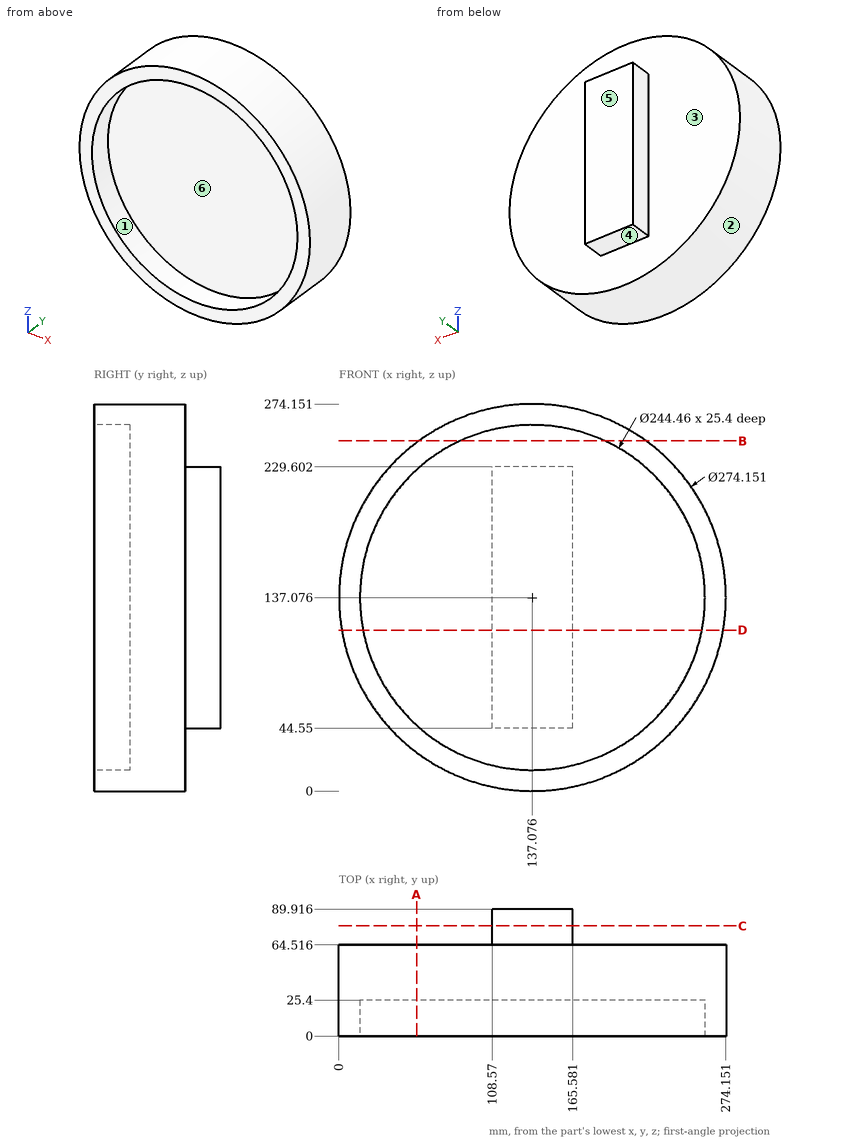
Verification items for this drawing (mm, ordinates from the low corner). A direction names the side the tool comes from. Coordinates: 2 decimals unless noted, no trailing zeros. Order: outer loops, then holes, each group sorted by start corner. A loop starts at its lowest first (then second) coordinate and runs counter-clockwise, first axis right, second up. Notation, with made-up numbers: (88.5, 44.5) - (112.5, 44.5) arc R32 ccw to (112.5, 72.5) - close; hole circle Ø6 at (4, -18.5). An arc over 180 degrees is marked (long way). Answer in a Markdown table with one row per item. Add a question column.
1. Material ranges on L1, parallel to X at y = 20.5, z = 141 (1 decimal); L2, parallel to Y at x = 125, z = 106; L3, parallel to X at y = 45, z = 134 (1 decimal), recorded low to high. Write a range as [from, to].
2. Section check C-C (y = 78). Enter the section's corners in (x, z), plus the area to 4 significant figures.
3. Access from +Z, -Z, +X, -X, +Y, -Y to the whole of each face (thin tool, end or side, straight path). Record for the marked faces 4, 5 and 6.
4. Section check B-B (z = 248). Enter the section's corners in (x, y) (1 decimal), plus the area to 3 significant figures.
5. Section check A-A (x = 55). Enter the section's corners in (y, z).
6. Section check D-D (z = 114). Enter the section's corners in (x, y) (1 decimal).
7. Gauge pin test, flat ends, axial feed: pin 1 Ø7.5 at (y, z) = (77, 148) entering from +X; pin 2 Ø10 at (x, z) = (65, 52) entering from +Y; pin 3 Ø6 at (x, y) = (217.5, 59) entering from -Z. Record the tip position at first contact, or that the pin passes through.
8. Draft check along Z on the marked faces 1, 2 and 3. Enter one of: +Z half, -Z half, draft (parallel to the pull), parting line (faces both ways), or undercut.
Data:
| question | item | result |
|---|---|---|
| 1 | L1 | x = [0.1, 14.9], [259.2, 274.1] |
| 1 | L2 | y = [25.4, 89.92] |
| 1 | L3 | x = [0, 274.1] |
| 2 | outline | (108.57, 44.55) - (165.58, 44.55) - (165.58, 229.6) - (108.57, 229.6) - close |
| 2 | area | 10,550 mm² |
| 3 | face 4 | -Z, +X, -X, +Y |
| 3 | face 5 | +Z, -Z, +X, -X, +Y |
| 3 | face 6 | -Y |
| 4 | outline | (56.5, 0) - (85.7, 0) - (85.7, 25.4) - (188.4, 25.4) - (188.4, 0) - (217.6, 0) - (217.6, 64.5) - (56.5, 64.5) - close |
| 4 | area | 7,780 mm² |
| 5 | outline | (0, 27.29) - (64.52, 27.29) - (64.52, 246.86) - (0, 246.86) - (0, 227.65) - (25.4, 227.65) - (25.4, 46.5) - (0, 46.5) - close |
| 6 | outline | (2, 0) - (17, 0) - (17, 25.4) - (257.1, 25.4) - (257.1, 0) - (272.2, 0) - (272.2, 64.5) - (165.6, 64.5) - (165.6, 89.9) - (108.6, 89.9) - (108.6, 64.5) - (2, 64.5) - close |
| 7 | pin 1 | stops at x = 165.58 |
| 7 | pin 2 | stops at y = 64.52 |
| 7 | pin 3 | stops at z = 23.96 |
| 8 | face 1 | undercut |
| 8 | face 2 | parting line |
| 8 | face 3 | draft |
